from build123d import *

# Parameters (mm, degrees)
SKETCH1_W             = 11.1125
SKETCH1_H             = 12.50125
BOSS_EXTRUDE1_DEPTH   = 2.54
SKETCH2_R             = 3.175
BOSS_EXTRUDE2_DEPTH   = 4.318
F_4_40_TAPPED_HOLE1_D = 2.2606


with BuildPart() as part:
    # Sketch1 → Boss-Extrude1 (new body)
    with BuildSketch(Plane(origin=(0, 0, 0), x_dir=(1, 0, 0), z_dir=(0, 1, 0))):
        with Locations((0, 16.881673618)):
            Rectangle(SKETCH1_W, SKETCH1_H)
    extrude(amount=BOSS_EXTRUDE1_DEPTH)

    # Sketch2 → Boss-Extrude2 (add)
    with BuildSketch(Plane(origin=(0, 2.54, 0), x_dir=(1, 0, 0), z_dir=(0, 1, 0))):
        with Locations(Location((0, 16.028548618, 0), (0, 0, 90))):
            Circle(SKETCH2_R)
    extrude(amount=BOSS_EXTRUDE2_DEPTH)

    # #4-40 Tapped Hole1 (through all)
    with Locations(Plane(origin=(0, 6.858, 0), x_dir=(-1, 0, 0), z_dir=(0, 1, 0))):
        with Locations((0, -16.028548618)):
            Hole(F_4_40_TAPPED_HOLE1_D / 2)


solid = part.part
The listing builds one solid part. Answer for the finished solid, in the listing's coordinates (mm). A direction names the side the tool comes from. Give positions to 0.01 mm unless a question says otherwise; leave off trailing zeros. Write each loop counter-clockwise with the first axis right and the second up, starting at its lowest first coordinate (ties: lowest second). Pieces come first, ordered by that corner, then holes.
1) Section C-C (y = 0.5) is taken. Write down the section's boundary in (x, z).
2) Find the intervals of material crossed by L1, parallel to Y at x = -3.25, z = -12.5; L2, parallel to Z at x = -0.25, y = 4.25; L3, parallel to X at y = 6, z = -18, in increasing order.
3) Section A-A (x = 0) is taken. Write down the section's boundary in (y, z), and give its area (3 significant figures).
4) For a pull along Z with two mould halves and no side action, classify faces 3 (the face through (-0.15, 3.38, -14.91)), 4 (the face through (0, 1, -10.631)), 5 (the face through (-1, 0, -17)), 6 (the face through (0, 1, -23.132)) as pulls with the +Z half, pulls with the -Z half, needs draft (parallel to the pull), parting line crosses it, or undercut.
5) Section B-B (z = -17) is taken. Write down the section's boundary in (x, y), and give its area (3 significant figures).
6) A tool of negligible diameter and unlimited length cuts with its end or side. For faces 1 (the face through (-5.556, 1, -17)), 2 (the face through (0, 2.54, -20)), from which of +Z, -Z, +X, -X, +Y, -Y can it reach the whole face along a straight path? Write none if from no direction.
7) Section D-D (x = 3.75) is taken. Write down the section's boundary in (y, z).
8) Given P1, Ø4, axis at x = -4, z = -17, coming from the +Y side; P2, Ø2, axis at x = 3.5, z = -13, coming from the +Y side, each flat-ended and moving along its own axis, determine where each tip first touches the part or whether it passes through.
Response:
1. outline: (-5.56, -23.13) - (5.56, -23.13) - (5.56, -10.63) - (-5.56, -10.63) - close; hole circle Ø2.26 at (0, -16.03)
2. L1: y = 0 to 2.54
2. L2: z = -19.19 to -17.13, -14.93 to -12.86
2. L3: x = -2.49 to 2.49
3. outline: (0, -23.13) - (2.54, -23.13) - (2.54, -19.2) - (6.86, -19.2) - (6.86, -17.16) - (0, -17.16) - close; (0, -14.9) - (6.86, -14.9) - (6.86, -12.85) - (2.54, -12.85) - (2.54, -10.63) - (0, -10.63) - close
3. area: 43.7 mm2
4. face 3: undercut
4. face 4: pulls with the +Z half
4. face 5: needs draft
4. face 6: pulls with the -Z half
5. outline: (-5.56, 0) - (-0.58, 0) - (-0.58, 6.86) - (-3.02, 6.86) - (-3.02, 2.54) - (-5.56, 2.54) - close; (0.58, 0) - (5.56, 0) - (5.56, 2.54) - (3.02, 2.54) - (3.02, 6.86) - (0.58, 6.86) - close
5. area: 46.4 mm2
6. face 1: +Z, -Z, -X, +Y, -Y
6. face 2: +Y
7. outline: (0, -23.13) - (2.54, -23.13) - (2.54, -10.63) - (0, -10.63) - close
8. P1: stops at y = 6.86
8. P2: stops at y = 2.54
